Can you work these out from the model? Positions are in its coordinate system, mm. Face numbers are marked on the shaded views. A direction names the side the tool comes from. Coordinates: 2 decimals unless noted, no trailing zeros. Write each loop counter-clockwise with the first axis right and the second up, starting at its lowest first coordinate (ties: lowest second). Pieces come first, ordered by that corner, then holes. Notation, with made-up numbers: (64, -3.5) -> (102, -3.5) arc R13 cw to (102, 20.5) -> close; hole circle Ø3 at (26, 87). An arc over 180 degrees is marked (long way). Use one line per item in the form item = value.
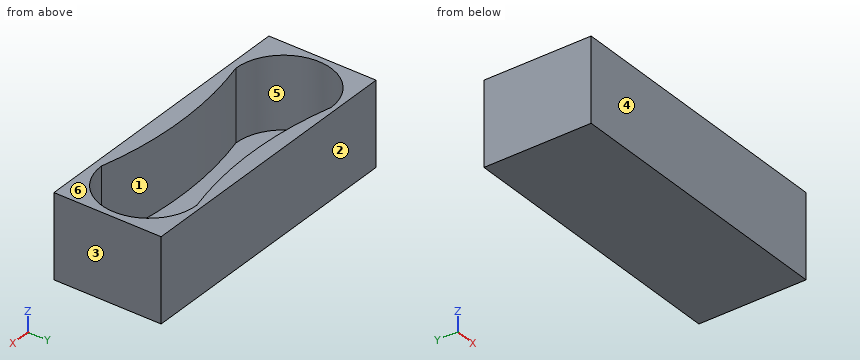
```python
from build123d import *

# Parameters (mm, degrees)
F0_W      = 240
F0_H      = 70
F1_DEPTH  = 45
F1_FACE_W = 240
F1_FACE_H = 70
F2_DEPTH  = 45
F5_DEPTH  = 60


with BuildPart() as f1:
    # F0 (on Front) → F1 (new body)
    with BuildSketch(Plane.XZ):
        Rectangle(F0_W, F0_H)
    extrude(amount=F1_DEPTH)

    # F1_face (on face) → F2 (join)
    with BuildSketch(Plane(origin=(0, 0, 0), x_dir=(1, 0, 0), z_dir=(0, 1, 0))):
        Rectangle(F1_FACE_W, F1_FACE_H)
    extrude(amount=F2_DEPTH)

    # F4 (on offset) → F5 (cut)
    with BuildSketch(Plane.XY.offset(35)):
        with BuildLine():
            ThreePointArc((-75.18201, -39.039491), (-0.18201, -29.513242), (74.81799, -39.039491))
            ThreePointArc((74.81799, -39.039491), (114.81799, 0.960509), (74.81799, 40.960509))
            ThreePointArc((74.81799, 40.960509), (-0.18201, 31.43426), (-75.18201, 40.960509))
            ThreePointArc((-75.18201, 40.960509), (-115.18201, 0.960509), (-75.18201, -39.039491))
        make_face()
    extrude(amount=-F5_DEPTH, mode=Mode.SUBTRACT)


solid = f1.part
```
Q1. Suppose I cut it at A-A (z = -16). Write out the boundary of the cut face in (x, y).
Return value:
outline = (-120, -45) -> (120, -45) -> (120, 45) -> (-120, 45) -> close; hole (-75.18, -39.04) arc R300 cw to (74.82, -39.04) arc R40 ccw to (74.82, 40.96) arc R300 cw to (-75.18, 40.96) arc R40 ccw to start
Q2. For the marked faces 5 and 6, which set-ups out of +Z, -Z, +X, -X, +Y, -Y let a thin tool reach every point of the face, with its end or its side?
Return value:
face_5 = +Z
face_6 = +Z, +X, -X, +Y, -Y
Q3. Suppose I cut it at C-C (x = 10). Write out the boundary of the cut face in (y, z).
Return value:
outline = (-45, -35) -> (45, -35) -> (45, 35) -> (31.61, 35) -> (31.61, -25) -> (-29.69, -25) -> (-29.69, 35) -> (-45, 35) -> close
Q4. Suppose I cut it at B-B (y = 3.5). Write out the boundary of the cut face in (x, z).
Return value:
outline = (-120, -35) -> (120, -35) -> (120, 35) -> (114.74, 35) -> (114.74, -25) -> (-115.1, -25) -> (-115.1, 35) -> (-120, 35) -> close
Q5. If I drill on line 1 (X direction, y = 2, z = -4); line 2 (Z direction, x = -8.5, y = -25); line 3 (X direction, y = -17.5, z = -16.5), over which ranges is the centre line in solid material (lowest first)? Write a range as from..to.
Return value:
line_1 = -120..-115.17, 114.8..120
line_2 = -35..-25
line_3 = -120..-110.67, 110.3..120
Q6. Will this pin go through, and if not, where does the flat tip stop? pin 1 (5 mm diameter, centred on x = -71, y = 14, fed in from +Z).
Return value:
pin_1 = -25
Q7. Thinking about a two-plate mould opening in Y: for the marked faces 1, 2, 3 and 4, which applies, released by +Y, released by -Y, zero draft, split by the parting line, or undercut?
Return value:
face_1 = undercut
face_2 = released by +Y
face_3 = zero draft
face_4 = released by -Y
